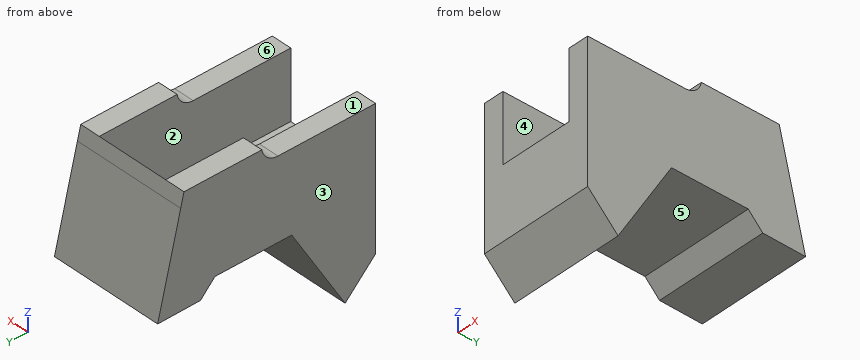
from build123d import *
from OCP.BRepFilletAPI import BRepFilletAPI_MakeChamfer

# Parameters (mm, degrees)
BOSS_EXTRUDE5_DEPTH = 14
SKETCH6_W           = 9
SKETCH6_H           = 23.591652045
CUT_EXTRUDE1_DEPTH  = 10
FILLET1_R           = 2
CHAMFER1_SIZE       = 10
CHAMFER1_SIZE2      = 7.296849953
CHAMFER1_SIZE2_2    = 7.289947028


with BuildPart() as part:
    # Sketch4 → Boss-Extrude5 (new body)
    with BuildSketch(Plane(origin=(0, 0, 0), x_dir=(0, 0, -1), z_dir=(1, 0, 0))):
        Polygon((-4.421768707, 9.149659864), (14.353741497, 13.707482993), (5.37414966, 4.927966044), (5.37414966, -4.527816269), (22.605249741, -14.850340136), (-4.421768707, -14.850340136), (-4.421768707, -0.850340136), (-6.10391849, -0.850340136), (-6.10391849, 8.741311909), align=None)
    extrude(amount=BOSS_EXTRUDE5_DEPTH)

    # Sketch6 → Cut-Extrude1 (cut)
    with BuildSketch(Plane.XY.offset(6.10391849)):
        with Locations((7, -3.054514114)):
            Rectangle(SKETCH6_W, SKETCH6_H)
    extrude(amount=-CUT_EXTRUDE1_DEPTH, mode=Mode.SUBTRACT)

    # Fillet1
    # the kernel refuses this fillet: 2 mm, written as the material it adds along each edge
    with BuildSketch(Plane(origin=(0, -0.850340136, 4.421768707), x_dir=(0, -1, 0), z_dir=(1, 0, 0))) as fillet1_piece_1:
        with BuildLine():
            CenterArc((1.974581282, -2), FILLET1_R, 90, 80.855488808)
            Line((0, -1.682149783), (-0.039491626, -1.675792779))
            ThreePointArc((-0.039491626, -1.675792779), (-0.04, -0.841074891), (-0.04, 0))
            Line((-0.04, 0), (0, 0.04))
            Line((0, 0.04), (1.974581282, 0.04))
            Line((1.974581282, 0.04), (1.974581282, 0))
        make_face()
    extrude(amount=2.5)
    with BuildSketch(Plane(origin=(11.5, -0.850340136, 4.421768707), x_dir=(0, 0, 1), z_dir=(1, 0, 0))) as fillet1_piece_2:
        with BuildLine():
            CenterArc((2, 1.974581282), FILLET1_R, 180, 80.855488808)
            Line((0, 1.974581282), (-0.04, 1.974581282))
            Line((-0.04, 1.974581282), (-0.04, 0))
            Line((-0.04, 0), (0, -0.04))
            ThreePointArc((0, -0.04), (0.841074891, -0.04), (1.675792779, -0.039491626))
            Line((1.675792779, -0.039491626), (1.682149783, 0))
        make_face()
    extrude(amount=2.5)

    # Chamfer1: one chamfer whose edges measure the first distance from different faces: ONE call of the kernel's chamfer builder (chamfer() names one face for all edges)
    chamfer1_edges_1 = [part.edges().sort_by_distance(p)[0] for p in [
        (7, 13.707482993, -14.353741497),
    ]]
    chamfer1_side_1 = [part.faces().sort_by_distance(p)[0] for p in [
        (7, 9.317724519, -9.863945578),
    ]]
    chamfer1_edges_2 = [part.edges().sort_by_distance(p)[0] for p in [
        (7, -14.850340136, -22.605249741),
    ]]
    chamfer1_side_2 = [part.faces().sort_by_distance(p)[0] for p in [
        (7, -14.850340136, -11.398988107),
    ]]
    chamfer1 = BRepFilletAPI_MakeChamfer(part.part.solid().wrapped)
    for e in chamfer1_edges_1:
        chamfer1.Add(CHAMFER1_SIZE, CHAMFER1_SIZE2, e.wrapped, chamfer1_side_1[0].wrapped)  # the first distance lies on this face
    for e in chamfer1_edges_2:
        chamfer1.Add(CHAMFER1_SIZE, CHAMFER1_SIZE2_2, e.wrapped, chamfer1_side_2[0].wrapped)  # the first distance lies on this face
    add(Compound.cast(chamfer1.Shape()), mode=Mode.REPLACE)


solid = part.part
Work out the finished part from the listing and answer in its coordinate system (mm). Face numbers are marked on the shaded views. A direction names the side the tool comes from. Give positions to 0.01 mm unless a question says otherwise; leave off trailing zeros. Write each loop counter-clockwise with the first axis right and the second up, starting at its lowest first coordinate (ties: lowest second). Pieces come first, ordered by that corner, then holes. Notation, with made-up numbers: M -1,75.5 L 41,75.5 A23 cw 41,98.5 Z; hole C -14,48.25 d5. An arc over 180 degrees is marked long. Answer as CSV lines item,"result".
Q1. Find the intervals of material crossed by probe 1 along X at (y, z) = (6.75, 3.5); probe 2 along Z at (x, y) = (4, -2); probe 3 along Z at (x, y) = (4.25, -11.25), in increasing order. Write a range as [from, to].
A:
probe 1,"x = [0, 2.5], [11.5, 14]"
probe 2,"z = [-5.37, -3.9]"
probe 3,"z = [-16.21, -3.9]"
Q2. A cutting plane is placed at A-A on x = 1.25. Write down the section's boundary in (y, z), plus the area to 3 significant figures.
A:
outline,"M -14.85,-12.61 L -11.1,-16.35 L -4.53,-5.37 L 4.93,-5.37 L 6.72,-7.2 L 11.99,-7.26 L 8.74,6.1 L -0.85,6.1 A2 cw -2.82,4.42 L -14.85,4.42 Z"
area,"345 mm²"
Q3. A cutting plane is placed at C-C on z = -3. Write down the section's boundary in (x, y), plus the area to 3 significant figures.
A:
outline,"M 0,-14.85 L 2.5,-14.85 L 2.5,8.74 L 11.5,8.74 L 11.5,-14.85 L 14,-14.85 L 14,10.95 L 0,10.95 Z"
area,"149 mm²"
Q4. The mould has two halves that part along X. Classify the marked faces 1, 2 and 3: +X half, -X half, draft (parallel to the pull), parting line (faces both ways), or undercut.
A:
face 1,"draft"
face 2,"undercut"
face 3,"-X half"
Q5. A tool of negligible diameter and unlimited length cuts with its end or side. For the marked faces 4, 5 and 6, from which of +Z, -Z, +X, -X, +Y, -Y can it reach the whole face along a straight path? Write none if from no direction.
A:
face 4,"+Z, -Y"
face 5,"-Z, +X, -X"
face 6,"+Z, +X, -X, -Y"
Q6. A cutting plane is placed at B-B on y = 1.5. Write down the section's boundary in (x, z), plus the area to 3 significant figures.
A:
outline,"M 0,-5.37 L 14,-5.37 L 14,6.1 L 11.5,6.1 L 11.5,-3.9 L 2.5,-3.9 L 2.5,6.1 L 0,6.1 Z"
area,"70.7 mm²"
Q7. Given P1, Ø8, axis at x = 10, y = -2.5, coming from the -Z side; P2, Ø2, axis at x = 13, y = -10.5, coming from the +Z side; P3, Ø4.5, axis at x = 5, z = 2.5, coming from the -Y side, each flat-ended and moving along its own axis, determine where each tip first touches the part or whether it passes through.
A:
P1,"stops at z = -8.67"
P2,"stops at z = 4.42"
P3,"stops at y = 8.74"
Q8. A cutting plane is placed at D-D on x = 9. Write down the section's boundary in (y, z).
A:
outline,"M -14.85,-12.61 L -11.1,-16.35 L -4.53,-5.37 L 4.93,-5.37 L 6.72,-7.2 L 11.99,-7.26 L 8.74,6.1 L 8.74,-3.9 L -14.85,-3.9 Z"
